from build123d import *

# Parameters (mm, degrees)
EXTRUDE_THIN1_DEPTH = 412.75
FILLET1_R           = 1.27


with BuildPart() as part:
    # Sketch1 → Extrude-Thin1 (new body)
    with BuildSketch(Plane.XY):
        with BuildLine():
            Line((0, 0), (-3.175, 0))
            ThreePointArc((-3.175, 0), (-3.728678916, 8.031723409), (-5.94070318, 15.772659394))
            ThreePointArc((-5.94070318, 15.772659394), (-8.027174826, 22.833539224), (-8.73125, 30.1625))
            Line((-8.73125, 30.1625), (-11.1125, 30.1625))
            Line((-11.1125, 30.1625), (-11.1125, 41.275))
            Line((-11.1125, 41.275), (0, 40.48125))
            Line((0, 40.48125), (-0.090483753, 39.214477451))
            Line((-0.090483753, 39.214477451), (-9.8425, 39.91105004))
            Line((-9.8425, 39.91105004), (-9.8425, 31.4325))
            Line((-9.8425, 31.4325), (-7.43958058, 31.4325))
            ThreePointArc((-7.43958058, 31.4325), (-6.895991056, 23.69982792), (-4.762762457, 16.247375785))
            ThreePointArc((-4.762762457, 16.247375785), (-2.59675891, 8.898174327), (-1.880316394, 1.27))
            Line((-1.880316394, 1.27), (0, 1.27))
            Line((0, 1.27), (0, 0))
        make_face()
    extrude(amount=-EXTRUDE_THIN1_DEPTH)

    # Fillet1
    fillet1_edges = [part.edges().sort_by_distance(p)[0] for p in [
        (-7.43958058, 31.4325, -206.375),
        (-3.175, 0, -206.375),
        (-11.1125, 30.1625, -206.375),
        (-11.1125, 41.275, -206.375),
    ]]
    fillet(fillet1_edges, radius=FILLET1_R)


solid = part.part
Verification items for the finished model (mm, model axes). A direction names the side the tool comes from. Round coordinates to 2 decimals unless told otherwise and drop trailing zeros. Loops run counter-clockwise (first coordinate to the right, second up) from the corner with the lowest first, then second, coordinate; pieces in that order, holes last. Notation, with made-up numbers: (88.5, 26.25) - (147.5, 26.25) arc R15 cw to (147.5, 44.25) - close; hole circle Ø10 at (26, 57). An arc over 180 degrees is marked (long way). Write item = value, one per line.
Q1. Mould release check, pull along Y, two halves, no side actions. Record for faces 4 (the flat face through (-4.944, 40.834, -203.486)), 5 (the cylindrical face through (-2.617, 9.004, -203.486)), 6 (the flat face through (-8, 24, -412.75)): +Y half, -Y half, draft (parallel to the pull), parting line (faces both ways), or undercut.
Here are the results:
face_4 = +Y half
face_5 = undercut
face_6 = draft
Q2. Sectioned sample at C-C on y = 26. Record the boundary of the cut face in (x, z), plus the area to 3 significant figures.
Here are the results:
outline = (-8.51, -412.75) - (-7.23, -412.75) - (-7.23, 0) - (-8.51, 0) - close
area = 527 mm^2
Q3. Tool access check on faces 1 (the flat face through (-8, 24, 0)), 2 (the cylindrical face through (-6.8, 23.17, -203.49)), 3 (the flat face through (-4.9, 39.56, -203.49)). Record the directions out of +Z, -Z, +X, -X, +Y, -Y that give a thin tool (end or side, any length) a straight path to the whole face; none if there is none.
Here are the results:
face_1 = +Z, +X, -X, +Y, -Y
face_2 = +Z, -Z, +X
face_3 = +Z, -Z
Q4. Sectioned sample at B-B on y = 6.5. Record the boundary of the cut face in (x, z), plus the area to 3 significant figures.
Here are the results:
outline = (-3.49, -412.75) - (-2.21, -412.75) - (-2.21, 0) - (-3.49, 0) - close
area = 529 mm^2
Q5. Material ranges on L1, parallel to Y at x = -9.75, z = -317; L2, parallel to X at y = 38.5, z = -151; L3, parallel to Y at x = -9, z = -162.5, recorded low to high.
Here are the results:
L1 = 30.16 to 31.43, 39.9 to 41.18
L2 = -11.11 to -9.84
L3 = 30.16 to 31.43, 39.85 to 41.12
Q6. Sectioned sample at A-A on z = -387. Record the boundary of the cut face in (x, y), plus the area to 3 significant figures.
Here are the results:
outline = (-11.11, 31.43) arc R1.27 ccw to (-9.84, 30.16) - (-8.73, 30.16) arc R38.5 ccw to (-5.94, 15.77) arc R38.5 cw to (-3.15, 1.27) arc R1.27 ccw to (-1.88, 0) - (0, 0) - (0, 1.27) - (-1.88, 1.27) arc R39.77 ccw to (-4.76, 16.25) arc R37.23 cw to (-7.46, 30.16) arc R1.27 ccw to (-8.73, 31.43) - (-9.84, 31.43) - (-9.84, 39.91) - (-0.09, 39.21) - (0, 40.48) - (-9.75, 41.18) arc R1.27 ccw to (-11.11, 39.91) - close
area = 69.7 mm^2
Q7. Depth check by flat-ended pin: pin 1 (6 mm diameter, centred on x = -8, z = -56.5, fed in from +Y); pin 2 (1.5 mm diameter, centred on x = -6.5, z = -206.5, fed in from +Y); pin 3 (2 mm diameter, centred on x = -1.5, z = -301, fed in from +Y); pin 4 (4 mm diameter, centred on y = 33.5, z = -270, fed in from +X). Enter the tip coordinate at first touch or a pass-through.
Here are the results:
pin_1 = 41.18
pin_2 = 41
pin_3 = 40.66
pin_4 = -9.84
